```python
from build123d import *

# Parameters (mm, degrees)
SKETCH1_W                = 140
SKETCH1_H                = 110
BOSS_EXTRUDE1_DEPTH      = 27
FILLET1_R                = 10
CUT_EXTRUDE1_DEPTH       = 25
CUT_EXTRUDE2_DEPTH       = 2
BOSS_EXTRUDE2_START      = 25
BOSS_EXTRUDE2_DEPTH      = 25
FILLET2_R                = 3
M3_CLEARANCE_HOLE1_D     = 3.4
M3_CLEARANCE_HOLE1_DEPTH = 15
M3_CLEARANCE_HOLE1_TIP   = 1.021463052
FILLET3_R                = 3


with BuildPart() as part:
    # Sketch1 → Boss-Extrude1 (new body)
    with BuildSketch(Plane.XY):
        with Locations((-49.99935, 35)):
            Rectangle(SKETCH1_W, SKETCH1_H)
    extrude(amount=BOSS_EXTRUDE1_DEPTH)

    # Fillet1
    fillet1_edges = [part.edges().sort_by_distance(p)[0] for p in [
        (20.00065, -20, 13.5),
        (-119.99935, -20, 13.5),
        (-119.99935, 90, 13.5),
        (20.00065, 90, 13.5),
    ]]
    fillet(fillet1_edges, radius=FILLET1_R)

    # Sketch3 → Cut-Extrude1 (cut)
    with BuildSketch(Plane(origin=(0, 0, 0), x_dir=(-1, 0, 0), z_dir=(0, 0, -1))):
        with BuildLine():
            Line((106.99935, 80), (-7.00065, 80))
            ThreePointArc((-7.00065, 80), (-9.121970344, 79.121320344), (-10.00065, 77))
            Line((-10.00065, 77), (-10.00065, -7))
            ThreePointArc((-10.00065, -7), (-9.121970344, -9.121320344), (-7.00065, -10))
            Line((-7.00065, -10), (106.99935, -10))
            ThreePointArc((106.99935, -10), (109.120670344, -9.121320344), (109.99935, -7))
            Line((109.99935, -7), (109.99935, 77))
            ThreePointArc((109.99935, 77), (109.120670344, 79.121320344), (106.99935, 80))
        make_face()
    extrude(amount=-CUT_EXTRUDE1_DEPTH, mode=Mode.SUBTRACT)

    # Sketch5 → Cut-Extrude2 (cut)
    with BuildSketch(Plane(origin=(0, 0, 0), x_dir=(-1, 0, 0), z_dir=(0, 0, -1))):
        with BuildLine():
            Line((-7.00065, -17), (106.99935, -17))
            ThreePointArc((106.99935, -17), (114.070417812, -14.071067812), (116.99935, -7))
            Line((116.99935, -7), (116.99935, 77))
            ThreePointArc((116.99935, 77), (114.070417812, 84.071067812), (106.99935, 87))
            Line((106.99935, 87), (-7.00065, 87))
            ThreePointArc((-7.00065, 87), (-14.071717812, 84.071067812), (-17.00065, 77))
            Line((-17.00065, 77), (-17.00065, -7))
            ThreePointArc((-17.00065, -7), (-14.071717812, -14.071067812), (-7.00065, -17))
        make_face()
        with BuildLine():
            Line((-7.00065, -13), (106.99935, -13))
            ThreePointArc((106.99935, -13), (111.241990687, -11.242640687), (112.99935, -7))
            Line((112.99935, -7), (112.99935, 77))
            ThreePointArc((112.99935, 77), (111.241990687, 81.242640687), (106.99935, 83))
            Line((106.99935, 83), (-7.00065, 83))
            ThreePointArc((-7.00065, 83), (-11.243290687, 81.242640687), (-13.00065, 77))
            Line((-13.00065, 77), (-13.00065, -7))
            ThreePointArc((-13.00065, -7), (-11.243290687, -11.242640687), (-7.00065, -13))
        make_face(mode=Mode.SUBTRACT)
    extrude(amount=-CUT_EXTRUDE2_DEPTH, mode=Mode.SUBTRACT)

    # Sketch6 → Boss-Extrude2 (add)
    with BuildSketch(Plane(origin=(0, 0, 25), x_dir=(-1, 0, 0), z_dir=(0, 0, -1)).offset(BOSS_EXTRUDE2_START)):
        with BuildLine():
            Line((0.862925656, 70.225224344), (0.862925656, 80))
            Line((0.862925656, 80), (-7.00065, 80))
            ThreePointArc((-7.00065, 80), (-9.121970344, 79.121320344), (-10.00065, 77))
            Line((-10.00065, 77), (-10.00065, 63.225224344))
            Line((-10.00065, 63.225224344), (-6.137074344, 63.225224344))
            ThreePointArc((-6.137074344, 63.225224344), (-1.187326876, 65.275476876), (0.862925656, 70.225224344))
        make_face()
        with BuildLine():
            Line((82.112925656, 70.225224344), (82.112925656, 80))
            Line((82.112925656, 80), (96.112925656, 80))
            Line((96.112925656, 80), (96.112925656, 70.225224344))
            ThreePointArc((96.112925656, 70.225224344), (89.112925656, 63.225224344), (82.112925656, 70.225224344))
        make_face()
        with BuildLine():
            Line((-10.00065, 12.453724344), (-10.00065, -1.546275656))
            Line((-10.00065, -1.546275656), (-10.00065, -7))
            ThreePointArc((-10.00065, -7), (-9.121970344, -9.121320344), (-7.00065, -10))
            Line((-7.00065, -10), (-4.00065, -10))
            Line((-4.00065, -10), (-4.00065, -1.211868999))
            ThreePointArc((-4.00065, -1.211868999), (0.777518707, 6.535585378), (-6.138374344, 12.453724344))
            Line((-6.138374344, 12.453724344), (-10.00065, 12.453724344))
        make_face()
        with BuildLine():
            Line((87.155325656, 12.175923879), (87.155325656, -1.265475191))
            ThreePointArc((87.155325656, -1.265475191), (96.112925656, 5.455224344), (87.155325656, 12.175923879))
        make_face()
        with BuildLine():
            Line((106.99935, 74), (109.99935, 74))
            Line((109.99935, 74), (109.99935, 77))
            ThreePointArc((109.99935, 77), (109.120670344, 79.121320344), (106.99935, 80))
            Line((106.99935, 80), (103.99935, 80))
            Line((103.99935, 80), (103.99935, 77))
            ThreePointArc((103.99935, 77), (104.878029656, 74.878679656), (106.99935, 74))
        make_face()
        with BuildLine():
            Line((103.99935, -7), (103.99935, -10))
            Line((103.99935, -10), (106.99935, -10))
            ThreePointArc((106.99935, -10), (109.120670344, -9.121320344), (109.99935, -7))
            Line((109.99935, -7), (109.99935, -4))
            Line((109.99935, -4), (106.99935, -4))
            ThreePointArc((106.99935, -4), (104.878029656, -4.878679656), (103.99935, -7))
        make_face()
    extrude(amount=-BOSS_EXTRUDE2_DEPTH)

    # Fillet2
    fillet2_edges = [part.edges().sort_by_distance(p)[0] for p in [
        (-0.862925656, 80, 12.5),
        (10.00065, 63.225224344, 12.5),
        (-96.112925656, 80, 12.5),
        (-82.112925656, 80, 12.5),
        (4.00065, -1.211868999, 12.5),
        (10.00065, 12.453724344, 12.5),
    ]]
    fillet(fillet2_edges, radius=FILLET2_R)

    # M3 Clearance Hole1
    with Locations(Plane(origin=(0, 0, 0), x_dir=(-1, 0, 0), z_dir=(0, 0, -1))):
        with Locations((-6.137074344, 70.225224344), (89.112925656, 70.225224344), (89.112925656, 5.455224344), (-6.138374344, 5.453724344), (-7.00065, 77), (106.99935, 77), (106.99935, -7), (-7.00065, -7)):
            Hole(M3_CLEARANCE_HOLE1_D / 2, depth=M3_CLEARANCE_HOLE1_DEPTH)
            with Locations((0, 0, -(M3_CLEARANCE_HOLE1_DEPTH + M3_CLEARANCE_HOLE1_TIP / 2))):  # 118° drill point
                Cone(0, M3_CLEARANCE_HOLE1_D / 2, M3_CLEARANCE_HOLE1_TIP, mode=Mode.SUBTRACT)

    # Fillet3
    fillet3_edges = [part.edges().sort_by_distance(p)[0] for p in [
        (-109.99935, 74, 12.5),
        (-103.99935, 80, 12.5),
        (-109.99935, -4, 12.5),
        (-103.99935, -10, 12.5),
        (4.00065, -10, 12.5),
    ]]
    fillet(fillet3_edges, radius=FILLET3_R - 0.0001)  # a hair under: the kernel refuses the full size


solid = part.part
```
Model file for the job. Use its own axes, mm. A direction names the side the tool comes from. Give positions to 0.01 mm unless a question says otherwise; leave off trailing zeros. Write each loop counter-clockwise with the first axis right and the second up, starting at its lowest first coordinate (ties: lowest second). Pieces come first, ordered by that corner, then holes. Notation, with made-up numbers: (73, 39.5) - (122, 39.5) arc R10 ccw to (122, 46.5) - close; hole circle Ø9 at (68.25, 74.5). An arc over 180 degrees is marked (long way). One line per question, with ' | ' between items. Start each with the question number.
(1) Slice it at B-B on x = -67. Write the cut outline in (y, z).
(2) Slice it at A-A on y = 33. Write the cut outline in (x, z).
(3) 3-axis set-ups, long thin cutter, end or side, ignore diameter. For faces 4 (the face through (-51, -20, 13)), 5 (the face through (-96.11, 5.27, 12.32)): which of +Z, -Z, +X, -X, +Y, -Y reach the whole face in a straight line?
(4) Slice it at C-C on z = 7.75. Give the number of separate pieces and of enclosed holes in the cut face, plus the area to 3 significant figures.
(5) Pin check, flat tip, straight feed: P1, Ø8, axis at x = -70, y = 7.5, coming from the -Z side. Stop position of the tip, or through.
(6) Wall check: line 1 along X through (y, z) = (-7, 4.5); line 2 along X through (y, z) = (53, 1.5); line 3 along X through (y, z) = (77, 5). Give the ranges that are in metal, low to high. Write a range as from..to.
(7) Two-plate mould, pull along Y, no slides. Class faces 1 (the face through (-51, 36, 27)), 2 (the face through (-96.97, 79.1, 12.68)), 3 (the face through (17.15, 86.99, 13.69)): +Y half, -Y half, draft (parallel to the pull), parting line (faces both ways), or undercut.
Results below:
1) outline: (-20, 0) - (-17, 0) - (-17, 2) - (-13, 2) - (-13, 0) - (-10, 0) - (-10, 25) - (80, 25) - (80, 0) - (83, 0) - (83, 2) - (87, 2) - (87, 0) - (90, 0) - (90, 27) - (-20, 27) - close
2) outline: (-120, 0) - (-117, 0) - (-117, 2) - (-113, 2) - (-113, 0) - (-110, 0) - (-110, 25) - (10, 25) - (10, 0) - (13, 0) - (13, 2) - (17, 2) - (17, 0) - (20, 0) - (20, 27) - (-120, 27) - close
3) face 4: +Z, -Z, +X, -X, -Y | face 5: -Z
4) separate pieces: 2 | enclosed holes: 9 | area: 5,200 mm^2
5) P1: z = 25
6) line 1: -120..-108.7, -105.3..-104, 4..5.3, 8.7..20 | line 2: -120..-117, -113..-110, 10..13, 17..20 | line 3: -120..-108.7, -105.3..-104, -96.11..-82.11, -0.86..5.3, 8.7..20
7) face 1: draft | face 2: undercut | face 3: +Y half
